from build123d import *

# Parameters (mm, degrees)
BOSS_EXTRUDE1_DEPTH = 19.05
CUT_EXTRUDE1_REACH  = 8.35
SKETCH6_W           = 1.778
SKETCH6_H           = 9.906
CUT_EXTRUDE2_DEPTH  = 50.8
SKETCH11_W          = 2.310054712
SKETCH11_H          = 0.25
CUT_EXTRUDE3_DEPTH  = 0.02
LPATTERN1_COUNT     = 7
LPATTERN1_PITCH     = 5.08
SKETCH13_W          = 2.286
SKETCH13_H          = 0.254
BOSS_EXTRUDE2_DEPTH = 0.02
LPATTERN2_COUNT     = 7
LPATTERN2_PITCH     = 5.08


with BuildPart() as part:
    # Sketch1 → Boss-Extrude1 (new body)
    with BuildSketch(Plane.XY):
        Polygon((0, 0), (19.05, 0), (19.05, 50.8), (12.7, 50.8), (12.7, 9.525), (0, 9.525), align=None)
    extrude(amount=BOSS_EXTRUDE1_DEPTH)

    # Sketch4 → Cut-Extrude1 (cut, up to next)
    with BuildSketch(Plane.ZY.offset(-12.7), mode=Mode.PRIVATE) as cut_extrude1_sk1:
        with BuildLine():
            Line((6.742001962, 13.600990631), (6.742001962, 46.700186434))
            ThreePointArc((6.742001962, 46.700186434), (9.525, 49.483184472), (12.307998038, 46.700186434))
            Line((12.307998038, 46.700186434), (12.307998038, 13.600990631))
            ThreePointArc((12.307998038, 13.600990631), (9.525, 10.817992593), (6.742001962, 13.600990631))
        make_face()
    cut_extrude1_tool1 = extrude(cut_extrude1_sk1.sketch, amount=-CUT_EXTRUDE1_REACH, mode=Mode.PRIVATE) & part.part
    add(cut_extrude1_tool1.solids().sort_by_distance((12.7, 30.150589, 9.525))[0], mode=Mode.SUBTRACT)

    # Sketch6 → Cut-Extrude2 (cut)
    with BuildSketch(Plane(origin=(0, 50.8, 0), x_dir=(1, 0, 0), z_dir=(0, 1, 0))):
        with Locations((18.161, -9.525)):
            Rectangle(SKETCH6_W, SKETCH6_H)
    extrude(amount=-CUT_EXTRUDE2_DEPTH, mode=Mode.SUBTRACT)

    # Sketch9 → CBORE for #8 Binding Head Machine Screw1 (revolve, cut)
    with BuildSketch(Plane(origin=(6.35, 9.525, 9.525), x_dir=(0, 0, 1), z_dir=(1, 0, 0))):
        Polygon((0, 0), (0, 9.525), (2.2479, 9.525), (2.2479, 2.667), (4.7625, 2.667), (4.7625, 0.532828266), (5.3975, 0), align=None)
    revolve(axis=Axis((6.35, 15.875, 9.525), (0, -1, 0)), mode=Mode.SUBTRACT)

    # Sketch11 → Cut-Extrude3 (cut)
    with BuildSketch(Plane.XY.offset(19.05)):
        with Locations((17.894972644, 42.293)):
            Rectangle(SKETCH11_W, SKETCH11_H)
    cut_extrude3 = extrude(amount=-CUT_EXTRUDE3_DEPTH, mode=Mode.SUBTRACT)

    # LPattern1: Cut-Extrude3 ×7
    with Locations(*[(0, -i * LPATTERN1_PITCH, 0) for i in range(1, LPATTERN1_COUNT)]):
        add(cut_extrude3, mode=Mode.SUBTRACT)

    # Sketch13 → Boss-Extrude2 (add)
    with BuildSketch(Plane(origin=(0, 0, 0), x_dir=(-1, 0, 0), z_dir=(0, 0, -1))):
        with Locations((-17.907, 41.749020167)):
            Rectangle(SKETCH13_W, SKETCH13_H)
    boss_extrude2 = extrude(amount=BOSS_EXTRUDE2_DEPTH)

    # LPattern2: Boss-Extrude2 ×7
    with Locations(*[(0, -i * LPATTERN2_PITCH, 0) for i in range(1, LPATTERN2_COUNT)]):
        add(boss_extrude2)


solid = part.part
Here's how the part is built. I have some questions about the finished solid (model axes, mm). A direction names the side the tool comes from. Coordinates: 2 decimals unless noted, no trailing zeros. Order: outer loops, then holes, each group sorted by start corner. A loop starts at its lowest first (then second) coordinate and runs counter-clockwise, first axis right, second up.
Item 1: If we section it at B-B on y = 28: List the corners of the cut face in (x, z) for me, plus the area to 3 significant figures.
Result sheet:
outline: (12.7, 0) - (19.05, 0) - (19.05, 4.57) - (17.27, 4.57) - (17.27, 6.74) - (12.7, 6.74) - close; (12.7, 12.31) - (17.27, 12.31) - (17.27, 14.48) - (19.05, 14.48) - (19.05, 19.05) - (12.7, 19.05) - close
area: 77.9 mm2
Item 2: If we section it at D-D on x = 15.5: List the corners of the cut face in (y, z) for me (3 decimals).
Result sheet:
outline: (0, 0) - (50.8, 0) - (50.8, 19.05) - (0, 19.05) - close; hole (13.601, 6.742) - (46.7, 6.742) arc R2.783 ccw to (46.7, 12.308) - (13.601, 12.308) arc R2.783 ccw to start
Item 3: For faces 5 (the face through (15, 30, 6.742)), 6 (the face through (17.272, 20, 13)), 7 (the face through (0.8, 9.525, 9.4)), 8 (the face through (7, 6.858, 7)), which set-ups out of +Z, -Z, +X, -X, +Y, -Y let a thin tool reach every point of the face, with its end or its side?
Result sheet:
face 5: +X, -X
face 6: +X, +Y, -Y
face 7: +Z, -Z, -X, +Y
face 8: +Y
Item 4: If we section it at C-C on y = 5.5: List the corners of the cut face in (x, z) for me (3 decimals), plus the area to 3 significant figures.
Result sheet:
outline: (0, 0) - (19.05, 0) - (19.05, 4.572) - (17.272, 4.572) - (17.272, 14.478) - (19.05, 14.478) - (19.05, 19.05) - (0, 19.05) - close; hole circle Ø4.496 at (6.35, 9.525)
area: 329 mm2
Item 5: If we mould it in two halves opening along X, with no side actions, what happens to faces 1 (the face through (7.21, 3.48, 11.6)), 2 (the face through (14, 20, 0)), 3 (the face through (1.628, 7.94, 8.905)), 4 (the face through (19.05, 25, 17))? For each: +X half, -X half, draft (parallel to the pull), parting line (faces both ways), or undercut.
Result sheet:
face 1: undercut
face 2: draft
face 3: undercut
face 4: +X half
Item 6: I need wall thicknesses on line 1 (Z direction, x = 6.35, y = 8.5); line 2 (X direction, y = 4, z = 9.5); line 3 (Z direction, x = 15, y = 3.5). Which ranges of each line are inside material? Lowest first, please.
Result sheet:
line 1: z = 0 to 4.76, 14.29 to 19.05
line 2: x = 0 to 4.1, 8.6 to 17.27
line 3: z = 0 to 19.05
Item 7: For P1, Ø4, axis at y = 45.5, z = 16.5, coming from the -X side, with a flat end and sliding along its axis, tell me the tip position at first contact or that it passes through.
Result sheet:
P1: stops at x = 12.7
